Input: dimensioned drawing with shaded views. Units: mm. Origin: part minimum x, y, z. A direction names the side the tool comes from. Coordinates: 2 decimals unless noted, no trailing zeros. Loops run counter-clockwise (first coordinate to the right, second up) from the corner with the lowest first, then second, coordinate; pieces in that order, holes last.
Item 1: Ray query, line 1 along Z through (x, y) = (56, 15.5) (1 decimal); line 2 along Z through (x, y) = (39.5, 15) (1 decimal); line 3 along X through (y, z) = (1.75, 9) (1 decimal). Return the intervals inside material, ascending.
Item 2: Reachability of the marked faces 1 and 2 from +Z, -Z, +X, -X, +Y, -Y: full face, straight path, thin tool, end or side. Return the list, or none.
Item 3: Section A-A on x = 16.5. Return loops of the section in (y, z).
Item 4: Contact query for flat-ended pins moving along their axis: P1, Ø8, axis at x = 43, z = 12.5, coming from the -Y side; P2, Ø4, axis at x = 23, y = 6, coming from the -Z side; P3, Ø2, axis at y = 3, z = 13.5, coming from the -X side (1 decimal); P4, Ø4, axis at x = 28, y = 7, coming from the -Z side. Output: stop coordinate, or through.
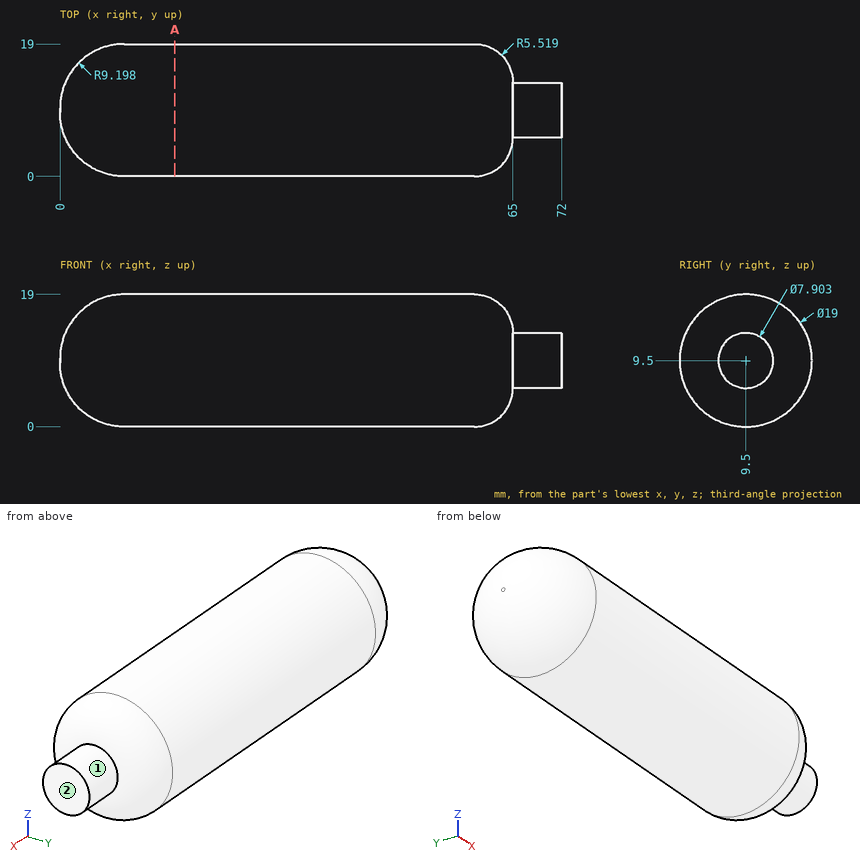
Results found:
1. line 1: z = 2.1 to 16.9
1. line 2: z = 1.8 to 17.2
1. line 3: x = 3.8 to 63.5
2. face 1: +X
2. face 2: +Z, -Z, +X, +Y, -Y
3. outline: circle Ø19 at (9.5, 9.5)
4. P1: stops at y = 0
4. P2: stops at z = 0.12
4. P3: stops at x = 2.5
4. P4: stops at z = 0.01
